For this review, take the finished solid that the model builds, in its own axes (mm). Face numbers are marked on the shaded views. A direction names the side the tool comes from. Round coordinates to 2 decimals unless told otherwise and drop trailing zeros. Loops run counter-clockwise (first coordinate to the right, second up) from the corner with the lowest first, then second, coordinate; pieces in that order, holes last.
1) Take a section at B-B (y = 11.5). State the section outline as (x, z) points, then the cut area to 3 significant figures.
2) Take a section at D-D (z = 30.5). State the section outline as (x, y) points.
3) Take a section at A-A (x = -17.5). State the section outline as (y, z) points, then the cut area to 3 significant figures.
4) Mouldability with a two-part tool opening along Z and no side actions: class the marked faces 4, 5 and 6 as pulls with the +Z half, pulls with the -Z half, needs draft (parallel to the pull), parting line crosses it, or undercut.
5) Wall thickness on L1, parallel to Y at x = -34.5, z = 22; L2, parallel to Y at x = 15, z = 16.5; L3, parallel to Y at x = -24, z = 29: over which ranges is each line inside the solid? List them lowest first.
6) Take a section at C-C (y = -16). State the section outline as (x, z) points, then the cut area to 3 significant figures.
7) Tool access review of the marked faces 1, 2 and 3: name each direction out of +Z, -Z, +X, -X, +Y, -Y from which nothing blocks a thin tool from reaching the whole face with its end or side.
8) Insertion check: pin 1 (1 mm diameter, centred on x = 24.5, z = 29, fed in from -Y). The pin has a flat end and moves straight along its axis. Give the tip position at first contact, or say it passes through.
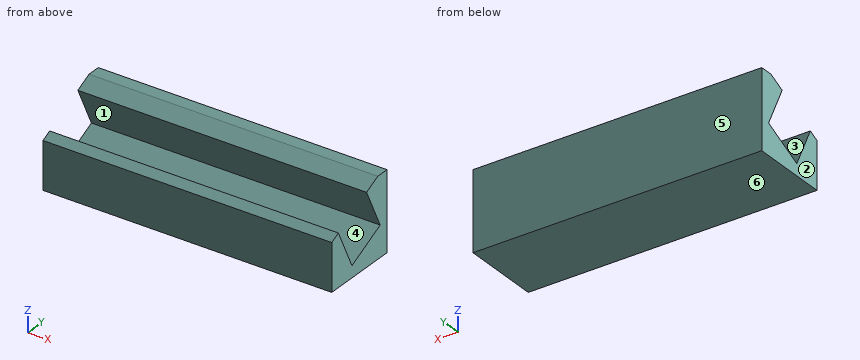
```python
from build123d import *

# Parameters (mm, degrees)
F0_W     = 139.7
F0_H     = 38.1
F1_DEPTH = 38.1
F3_DEPTH = 139.701
F5_DEPTH = 139.701


with BuildPart() as f1:
    # F0 (on Top) → F1 (new body)
    with BuildSketch(Plane.XY):
        Rectangle(F0_W, F0_H)
    extrude(amount=F1_DEPTH)

    # F2 (on face) → F3 (cut, through all)
    with BuildSketch(Plane.YZ.offset(69.85)):
        Polygon((-19.05, 22.86), (12.7, 38.1), (-19.05, 38.1), align=None)
    extrude(amount=-F3_DEPTH, mode=Mode.SUBTRACT)

    # F4 (on face) → F5 (cut, through all)
    with BuildSketch(Plane.YZ.offset(69.85)):
        Polygon((14.336284, 14.937055), (4.99362, 34.400938), (-14.470263, 25.058274), (-5.127599, 5.594391), align=None)
    extrude(amount=-F5_DEPTH, mode=Mode.SUBTRACT)


solid = f1.part
```
Response:
1. outline: (-69.85, 0) - (69.85, 0) - (69.85, 13.58) - (-69.85, 13.58) - close; (-69.85, 20.85) - (69.85, 20.85) - (69.85, 37.52) - (-69.85, 37.52) - close
1. area: 4,230 mm2
2. outline: (-69.85, 6.87) - (69.85, 6.87) - (69.85, 19.05) - (-69.85, 19.05) - close
3. outline: (-19.05, 0) - (19.05, 0) - (19.05, 38.1) - (12.7, 38.1) - (4.99, 34.4) - (14.34, 14.94) - (-5.13, 5.59) - (-14.47, 25.06) - (-19.05, 22.86) - close
3. area: 744 mm2
4. face 4: undercut
4. face 5: needs draft
4. face 6: pulls with the -Z half
5. L1: y = -19.05 to -13, 10.95 to 19.05
5. L2: y = -19.05 to -10.36, 13.59 to 19.05
5. L3: y = 7.59 to 19.05
6. outline: (-69.85, 0) - (69.85, 0) - (69.85, 24.32) - (-69.85, 24.32) - close
6. area: 3,400 mm2
7. face 1: +X, -X
7. face 2: +Z, -Z, -X, +Y, -Y
7. face 3: +Z, +X, -X
8. pin 1: stops at y = 7.35
